Part print with two shaded views. Sizes in mm from the minimum x, y, z corner. Give positions to 0.01 mm unless a question says otherwise; leave off trailing zeros. Loops run counter-clockwise (first coordinate to the right, second up) from the corner with the lowest first, then second, coordinate; pieces in that order, holes last. Notation, with made-up numbers: M 44,81 L 82,81 A25 cw 82,105 Z; hole C 51,81.5 d2. An arc over 180 degrees is marked long. Answer as a JSON object with one key per item and string values. Group by question number.
1. Slice it at C-C (y = 3.15). List the corners of the cut face in (x, z).
2. Drop flat-ended pins along their axis: pin 1 Ø3.5 at (x, z) = (6.5, 5) entering from -Y; pin 2 Ø5 at (x, z) = (15, 1.5) entering from -Y. Give the stop position or say it passes through.
3. Mould opens along X. For the marked faces 1, 2 and 3 say: released by +X, released by -X, zero draft, split by the parting line, or undercut.
4. Slice it at D-D (z = 4). List the corners of the cut face in (x, y), then the cut area to 3 significant figures.
5. Slice it at A-A (x = 6.5). List the corners of the cut face in (y, z), then the cut area to 3 significant figures.
6. Drill centre lines: line 1 along Z through (x, y) = (6.5, 2.25); line 2 along X through (y, z) = (1.35, 4.75); line 3 along X through (y, z) = (1.65, 4.5). Where is each one in solid material? Low to high. Write a range as [from, to].
7. Slice it at B-B (z = 5). List the corners of the cut face in (x, y).
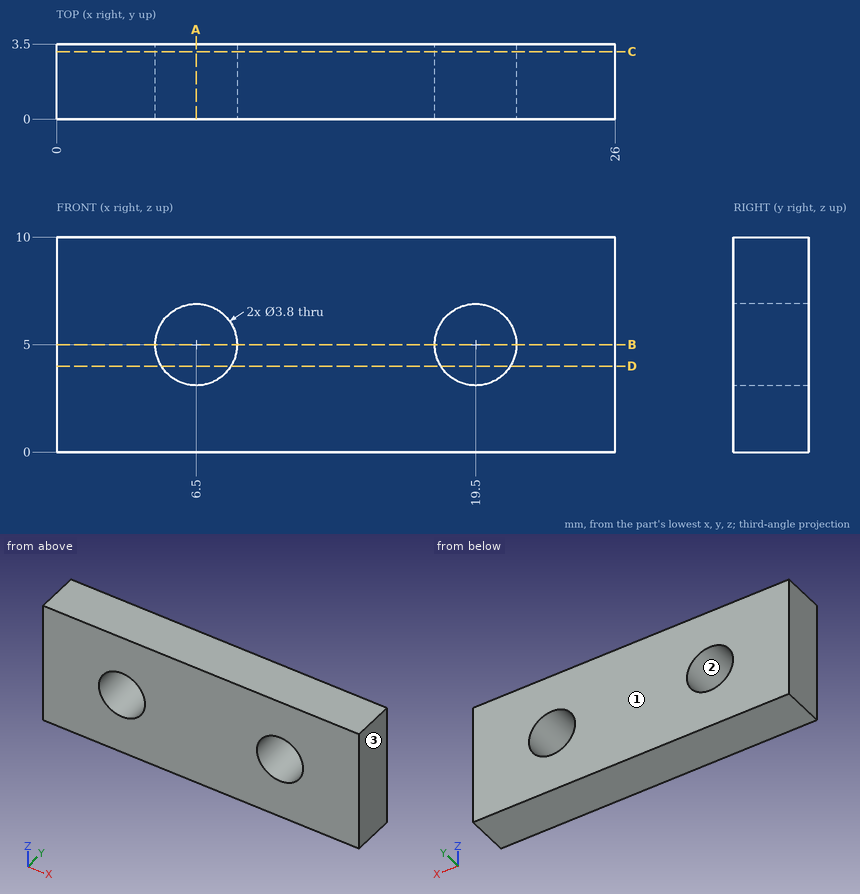
Established:
{
 "1": {"outline": "M 0,0 L 26,0 L 26,10 L 0,10 Z; hole C 6.5,5 d3.8; hole C 19.5,5 d3.8"},
 "2": {"pin 1": "passes through", "pin 2": "stops at y = 0"},
 "3": {"face 1": "zero draft", "face 2": "undercut", "face 3": "released by +X"},
 "4": {"outline": "M 0,0 L 4.88,0 L 4.88,3.5 L 0,3.5 Z; M 8.12,0 L 17.88,0 L 17.88,3.5 L 8.12,3.5 Z; M 21.12,0 L 26,0 L 26,3.5 L 21.12,3.5 Z", "area": "68.4 mm^2"},
 "5": {"outline": "M 0,0 L 3.5,0 L 3.5,3.1 L 0,3.1 Z; M 0,6.9 L 3.5,6.9 L 3.5,10 L 0,10 Z", "area": "21.7 mm^2"},
 "6": {"line 1": "z = [0, 3.1], [6.9, 10]", "line 2": "x = [0, 4.62], [8.38, 17.62], [21.38, 26]", "line 3": "x = [0, 4.67], [8.33, 17.67], [21.33, 26]"},
 "7": {"outline": "M 0,0 L 4.6,0 L 4.6,3.5 L 0,3.5 Z; M 8.4,0 L 17.6,0 L 17.6,3.5 L 8.4,3.5 Z; M 21.4,0 L 26,0 L 26,3.5 L 21.4,3.5 Z"}
}
